Read the model definition and answer for the solid it produces. Units are mm, in the model's axes. Give positions to 0.01 mm unless a question says otherwise; leave off trailing zeros. Write each loop counter-clockwise with the first axis right and the second up, starting at its lowest first coordinate (ties: lowest second). Pieces come first, ordered by that corner, then holes. Notation, with made-up numbers: M -16.5,-38 L 3.5,-38 A16 cw 3.5,-7 Z; hole C -20.75,-13 d6. An arc over 180 degrees is marked long. Answer as CSV lines item,"result". Start each with the question number.
Autodesk Fusion 360 part; units mm, degrees
sketch "Sketch1" plane through (0, 0, 0) normal (0, 0, 1) x (1, 0, 0)
  circle A0 centre (0, 0) radius 25
  dimension "d1" = 50
extrude "Extrude1" add sketch "Sketch1" along normal blind 5
sketch "Sketch2" plane through (0, 0, 5) normal (0, 0, 1) x (-1, 0, 0)
  circle A0 centre (0, 0) radius 25
  circle A1 centre (0, 0) radius 12.5
  dimension "d4" = 25
extrude "Extrude2" add sketch "Sketch2" along normal blind 550 contours A1
sketch "Sketch3" plane through (0, 0, 555) normal (0, 0, 1) x (-1, 0, 0)
  circle A0 centre (0, 0) radius 12.5
  line L0 (0, -5) -> (-100, -5)
  line L1 (-100, -5) -> (-100, 5)
  line L2 (-100, 5) -> (0, 5)
  line L3 (0, 5) -> (0, -5)
  dimension "d7" = 100
  dimension "d8" = 10
extrude "Extrude3" add sketch "Sketch3" against normal blind 525 contours A0 L0 L1 L2
extrude "Extrude4" cut sketch "Sketch3" against normal blind 25 contours A0 L0 L1 L2
sketch "Sketch4" plane through (0, 0, 555) normal (0, 0, 1) x (-1, 0, 0)
  circle A0 centre (0, 0) radius 12.5
  circle A1 centre (0, 0) radius 3
  dimension "d13" = 6
extrude "Extrude5" cut sketch "Sketch4" against normal blind 10 contours A1
extrude "Extrude6" cut 1 faces at (70.8333, 0, 530) along direction (0, 0, -1) blind 5
extrude "Extrude7" cut 1 faces at (70.8333, 0, 30) along direction (0, 0, 1) blind 5
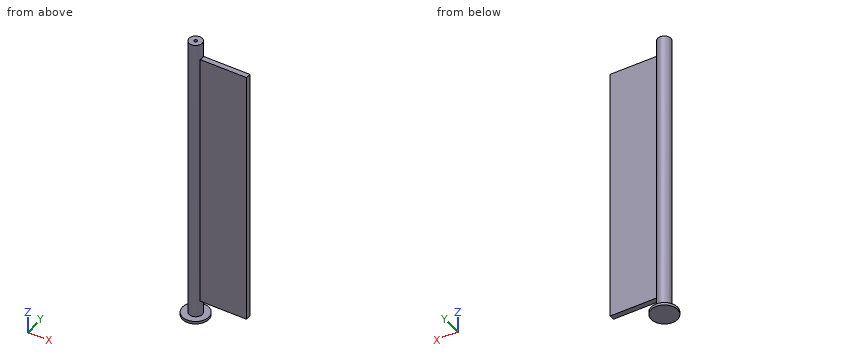
1. Find section A-A on z = 447.5. Determine the outline of the cut face in (x, y).
2. Find section B-B on x = 68. Determine the outline of the cut face in (y, z).
3. Find the intervals of material crossed by line 1 (Y direction, x = 0, z = 547); line 2 (Y direction, x = 52.5, z = 155.5), in increasing order. Write a range as [from, to].
4. Given pin 1 (12 mm diameter, centred on y = 15, z = 411.5, fed in from -X); pin 2 (8 mm diameter, centred on x = 63, y = -0.5, fed in from -Z); pin 3 (6 mm diameter, centred on y = 16, z = 430, fed in from +X); pin 4 (1 mm diameter, centred on x = 12.5, z = 372.5, fed in from +Y), each flat-ended and moving along its own axis, determine where each tip first touches the part or whether it passes through.
Computed:
1,outline,"M 11.46,-5 L 100,-5 L 100,5 L 11.46,5 A12.5 ccw long Z"
2,outline,"M -5,35 L 5,35 L 5,525 L -5,525 Z"
3,line 1,"y = [-12.5, -3], [3, 12.5]"
3,line 2,"y = [-5, 5]"
4,pin 1,"stops at x = -8.67"
4,pin 2,"stops at z = 35"
4,pin 3,"passes through"
4,pin 4,"stops at y = 5"
